```python
from build123d import *

# Parameters (mm, degrees)
EXTRUDE_1_OUTLINE_R = 1.7
EXTRUDE_1_DEPTH     = 3
FILLET_1_R          = 3
FILLET_2_R          = 5
SKETCH_2_R          = 3.5
EXTRUDE_2_DEPTH     = 7
CHAMFER_1_SIZE      = 4
CHAMFER_1_SIZE2     = 3.356398525
SKETCH_3_R          = 1.6
CUT_EXTRUDE_1_DEPTH = 50
CUT_EXTRUDE_2_DEPTH = 1.2
CUT_EXTRUDE_3_DEPTH = 10
FILLET_3_R          = 5
EXTRUDE_START       = -10
SKETCH_6_R          = 2.5
SKETCH_6_R_2        = 1.5
EXTRUDE_1_2_DEPTH   = 10


# Read off the part's stored shape, not the designer's step: 보스-돌출1
with BuildPart() as part:
    # Extrude 1 outline → Extrude 1 (new body)
    with BuildSketch(Plane.XY):
        Polygon((61.805886205, -13.571810541), (61.805886205, 6.428189459), (17.805886205, 6.428189459), (17.805886205, 21.428189459), (-12.194113795, 21.428189459), (-12.194113795, 29.428189459), (17.805886205, 29.428189459), (17.805886205, 105.728189459), (-106.694113795, 105.728189459), (-106.694113795, 29.428189459), (-76.694113795, 29.428189459), (-76.694113795, 21.428189459), (-106.694113795, 21.428189459), (-106.694113795, 0.157968071), (-2.194113795, -0.252198443), (-2.194113795, -13.571810541), align=None)
        with Locations((-98.694113795, 13.428189459)):
            Circle(EXTRUDE_1_OUTLINE_R, mode=Mode.SUBTRACT)
        with Locations((2.805886205, -8.571810541)):
            Circle(EXTRUDE_1_OUTLINE_R, mode=Mode.SUBTRACT)
        with Locations((2.805886205, 1.428189459)):
            Circle(EXTRUDE_1_OUTLINE_R, mode=Mode.SUBTRACT)
        with Locations((2.805886205, 13.428189459)):
            Circle(EXTRUDE_1_OUTLINE_R, mode=Mode.SUBTRACT)
        with Locations((56.805886205, -8.979991995)):
            Circle(EXTRUDE_1_OUTLINE_R, mode=Mode.SUBTRACT)
        with Locations((56.805886205, 1.428189459)):
            Circle(EXTRUDE_1_OUTLINE_R, mode=Mode.SUBTRACT)
        with Locations((-98.694113795, 89.428189459)):
            Circle(EXTRUDE_1_OUTLINE_R, mode=Mode.SUBTRACT)
        with Locations((2.805886205, 89.428189459)):
            Circle(EXTRUDE_1_OUTLINE_R, mode=Mode.SUBTRACT)
    extrude(amount=EXTRUDE_1_DEPTH)

    # 필렛1
    fillet_1_edges = [part.edges().sort_by_distance(p)[0] for p in [
        (-76.694113795, 21.428189459, 1.5),
        (-76.694113795, 29.428189459, 1.5),
        (-12.194113795, 29.428189459, 1.5),
        (-12.194113795, 21.428189459, 1.5),
    ]]
    fillet(fillet_1_edges, radius=FILLET_1_R)

    # 필렛2
    fillet_2_edges = [part.edges().sort_by_distance(p)[0] for p in [
        (61.805886205, 6.428189459, 1.5),
        (61.805886205, -13.571810541, 1.5),
        (-2.194113795, -13.571810541, 1.5),
        (-2.194113795, -0.252198443, 1.5),
        (-106.694113795, 0.157968071, 1.5),
        (-106.694113795, 21.428189459, 1.5),
        (-106.694113795, 29.428189459, 1.5),
        (-106.694113795, 105.728189459, 1.5),
        (17.805886205, 105.728189459, 1.5),
        (17.805886205, 29.428189459, 1.5),
        (17.805886205, 21.428189459, 1.5),
        (17.805886205, 6.428189459, 1.5),
    ]]
    fillet(fillet_2_edges, radius=FILLET_2_R)

    # 스케치2 → 보스-돌출2 (add)
    with BuildSketch(Plane.XY.offset(3)):
        with Locations((-98.694113795, 89.428189459)):
            Circle(SKETCH_2_R)
        with Locations((2.805886205, 89.428189459)):
            Circle(SKETCH_2_R)
        with Locations((-98.694113795, 13.428189459)):
            Circle(SKETCH_2_R)
        with Locations((2.805886205, 13.428189459)):
            Circle(SKETCH_2_R)
    extrude(amount=EXTRUDE_2_DEPTH)

    # 모따기1
    chamfer_1_edges = [part.edges().sort_by_distance(p)[0] for p in [
        (-102.194113795, 89.428189459, 3),
        (-0.694113795, 89.428189459, 3),
        (-102.194113795, 13.428189459, 3),
        (-0.694113795, 13.428189459, 3),
    ]]
    chamfer_1_side = [part.faces().sort_by_distance(p)[0] for p in [
        (-38.126255905, 49.180268575, 3),
    ]]
    chamfer(chamfer_1_edges, length=CHAMFER_1_SIZE, length2=CHAMFER_1_SIZE2, reference=chamfer_1_side[0])

    # 스케치3 → 컷-돌출1 (cut)
    with BuildSketch(Plane(origin=(0, 0, 0), x_dir=(-1, 0, 0), z_dir=(0, 0, -1))):
        with Locations(Location((-2.805886205, 89.428189459, 0), (0, 0, 180))):
            Circle(SKETCH_3_R)
        with Locations(Location((-2.805886205, 13.428189459, 0), (0, 0, 180))):
            Circle(SKETCH_3_R)
        with Locations(Location((98.694113795, 13.428189459, 0), (0, 0, 180))):
            Circle(SKETCH_3_R)
        with Locations(Location((98.694113795, 89.428189459, 0), (0, 0, 180))):
            Circle(SKETCH_3_R)
    extrude(amount=-CUT_EXTRUDE_1_DEPTH, mode=Mode.SUBTRACT)

    # 스케치4 → 컷-돌출2 (cut)
    with BuildSketch(Plane.XY.offset(3)):
        Polygon((6.039047712, 1.428189459), (4.422466959, 4.228189459), (1.189305451, 4.228189459), (-0.427275303, 1.428189459), (1.189305451, -1.371810541), (4.422466959, -1.371810541), align=None)
        Polygon((6.039047712, -8.571810541), (4.422466959, -5.771810541), (1.189305451, -5.771810541), (-0.427275303, -8.571810541), (1.189305451, -11.371810541), (4.422466959, -11.371810541), align=None)
        Polygon((53.572724697, 1.428189459), (55.189305451, -1.371810541), (58.422466959, -1.371810541), (60.039047712, 1.428189459), (58.422466959, 4.228189459), (55.189305451, 4.228189459), align=None)
        Polygon((53.572724697, -8.979991995), (55.189305451, -11.779991995), (58.422466959, -11.779991995), (60.039047712, -8.979991995), (58.422466959, -6.179991995), (55.189305451, -6.179991995), align=None)
    extrude(amount=-CUT_EXTRUDE_2_DEPTH, mode=Mode.SUBTRACT)

    # 스케치5 → 컷-돌출3 (cut)
    with BuildSketch(Plane.XY.offset(3)):
        Polygon((-44.444113795, 90.728189459), (-44.444113795, 52.86409473), (-34.510431855, 44.428189459), (-19.444113795, 44.428189459), (-19.444113795, 90.728189459), align=None)
        Polygon((-69.444113795, 90.728189459), (-69.444113795, 74.094654862), (-44.444113795, 52.86409473), (-44.444113795, 90.728189459), align=None)
        Polygon((-44.444113795, 52.86409473), (-69.444113795, 74.094654862), (-69.444113795, 44.428189459), (-34.510431855, 44.428189459), align=None)
    extrude(amount=-CUT_EXTRUDE_3_DEPTH, mode=Mode.SUBTRACT)

    # 필렛3
    fillet_3_edges = [part.edges().sort_by_distance(p)[0] for p in [
        (-19.444113795, 90.728189459, 1.5),
        (-19.444113795, 44.428189459, 1.5),
        (-69.444113795, 44.428189459, 1.5),
        (-69.444113795, 90.728189459, 1.5),
    ]]
    fillet(fillet_3_edges, radius=FILLET_3_R)

    # 스케치6 → Extrude 1 2 (add)
    # profile 1 of 4: a face of its own
    with BuildSketch(Plane(origin=(0, 0, 0), x_dir=(-1, 0, 0), z_dir=(0, 0, -1)).offset(EXTRUDE_START)):
        with Locations((-2.805886205, 89.428189459)):
            Circle(SKETCH_6_R)
        with Locations((-2.805886205, 89.428189459)):
            Circle(SKETCH_6_R_2, mode=Mode.SUBTRACT)
    # profile 2 of 4: a face of its own
    with BuildSketch(Plane(origin=(0, 0, 0), x_dir=(-1, 0, 0), z_dir=(0, 0, -1)).offset(EXTRUDE_START)):
        with Locations((-2.805886205, 13.428189459)):
            Circle(SKETCH_6_R)
        with Locations((-2.805886205, 13.428189459)):
            Circle(SKETCH_6_R_2, mode=Mode.SUBTRACT)
    # profile 3 of 4: a face of its own
    with BuildSketch(Plane(origin=(0, 0, 0), x_dir=(-1, 0, 0), z_dir=(0, 0, -1)).offset(EXTRUDE_START)):
        with Locations((98.694113795, 13.428189459)):
            Circle(SKETCH_6_R)
        with Locations((98.694113795, 13.428189459)):
            Circle(SKETCH_6_R_2, mode=Mode.SUBTRACT)
    # profile 4 of 4: a face of its own
    with BuildSketch(Plane(origin=(0, 0, 0), x_dir=(-1, 0, 0), z_dir=(0, 0, -1)).offset(EXTRUDE_START)):
        with Locations((98.694113795, 89.428189459)):
            Circle(SKETCH_6_R)
        with Locations((98.694113795, 89.428189459)):
            Circle(SKETCH_6_R_2, mode=Mode.SUBTRACT)
    extrude(amount=EXTRUDE_1_2_DEPTH)


solid = part.part
```
Geometry check sheet. Reference: the model listing, model coordinates, mm. A direction names the side the tool comes from. Round coordinates to 2 decimals unless told otherwise and drop trailing zeros. Loops run counter-clockwise (first coordinate to the right, second up) from the corner with the lowest first, then second, coordinate; pieces in that order, holes last. Notation, with made-up numbers: (15, -29) -> (29, -29) arc R29 cw to (29, -8) -> close; hole circle Ø10 at (61, 44.5). An arc over 180 degrees is marked (long way). Use a Markdown table: item, result.
(1) Go/stop test with flat-tipped pins: P1, Ø5, axis at x = -98.69, y = 89.43, coming from the -Z side; P2, Ø4.5, axis at x = 56.5, y = -10, coming from the +Z side; P3, Ø0.9, axis at x = -44.5, z = 1, coming from the -Y side; P4, Ø2.5, axis at y = 80, z = 2, coming from the +X side. Record where each tip stops, or that it passes through.
Calculated:
| item | result |
|---|---|
| P1 | z = 0 |
| P2 | z = 3 |
| P3 | y = -0.09 |
| P4 | x = 17.81 |
(2) Sectioned sample at C-C (z = 4.75). Enter the section's corners in (x, y), then the cut area to 3 significant figures.
Calculated:
| item | result |
|---|---|
| outline | circle Ø10.83 at (-98.69, 13.43); circle Ø10.83 at (-98.69, 89.43); circle Ø10.83 at (2.81, 13.43); circle Ø10.83 at (2.81, 89.43); hole circle Ø3 at (-98.69, 13.43); hole circle Ø3 at (-98.69, 89.43); hole circle Ø3 at (2.81, 13.43); hole circle Ø3 at (2.81, 89.43) |
| area | 340 mm² |
(3) Sectioned sample at D-D (x = 47). Enter the section's corners in (y, z), then the cut area to 3 significant figures.
Calculated:
| item | result |
|---|---|
| outline | (-13.57, 0) -> (6.43, 0) -> (6.43, 3) -> (-13.57, 3) -> close |
| area | 60.0 mm² |
(4) Mould release check, pull along X, two halves, no side actions. Record for faces 1 (the cylindrical face through (16.302, 20.002, 1.521)), 2 (the cylindrical face through (-20.9, 45.9, 1.5)), 3 (the cylindrical face through (-105.268, 19.925, 1.521)): released by +X, released by -X, zero draft, split by the parting line, or undercut.
Calculated:
| item | result |
|---|---|
| face 1 | released by +X |
| face 2 | undercut |
| face 3 | released by -X |
(5) Sectioned sample at B-B (x = -83). Enter the section's corners in (y, z).
Calculated:
| item | result |
|---|---|
| outline | (0.06, 0) -> (21.43, 0) -> (21.43, 3) -> (0.06, 3) -> close; (29.43, 0) -> (105.73, 0) -> (105.73, 3) -> (29.43, 3) -> close |
(6) Sectioned sample at A-A (y = 72). Enter the section's corners in (x, z), then the cut area to 4 significant figures.
Calculated:
| item | result |
|---|---|
| outline | (-106.69, 0) -> (-69.44, 0) -> (-69.44, 3) -> (-106.69, 3) -> close; (-19.44, 0) -> (17.81, 0) -> (17.81, 3) -> (-19.44, 3) -> close |
| area | 223.5 mm² |
(7) Set-up check for faces 4 (the cylindrical face through (6.144, 90.479, 8.153)), 5 (the cylindrical face through (-68.018, 45.932, 1.479)), 6 (the cylindrical face through (19.232, 7.932, 1.521)): record each of +Z, -Z, +X, -X, +Y, -Y from which the full face is reachable in a straight line by a thin tool's end or side.
Calculated:
| item | result |
|---|---|
| face 4 | +Z |
| face 5 | +Z, -Z |
| face 6 | +Z, -Z, +X, +Y |
(8) Scan lines: probe 1 along X at (y, z) = (89.5, 9.25); probe 2 along X at (y, z) = (54, 2.75); probe 3 along X at (y, z) = (13, 7). Record each from-to range of solid material in increasing order.
Calculated:
| item | result |
|---|---|
| probe 1 | -102.19 to -100.19, -97.2 to -95.19, -0.69 to 1.31, 4.3 to 6.31 |
| probe 2 | -106.69 to -69.44, -19.44 to 17.81 |
| probe 3 | -102.17 to -100.13, -97.26 to -95.22, -0.67 to 1.37, 4.24 to 6.28 |
